from build123d import *

# Parameters (mm, degrees)
SKETCH1_R           = 3.175
BOSS_EXTRUDE1_DEPTH = 1.5875
FILLET1_R           = 9.525


with BuildPart() as part:
    # Sketch1 → Boss-Extrude1 (new body)
    with BuildSketch(Plane(origin=(0, 0, 0), x_dir=(1, 0, 0), z_dir=(0, 1, 0))):
        Polygon((12.7, 12.7), (14.2875, 12.7), (20.6375, 12.7), (22.225, 12.7), (47.625, 12.7), (47.625, -12.7), (22.225, -12.7), (12.7, -12.7), (-12.7, -12.7), (-22.225, -12.7), (-47.625, -12.7), (-47.625, 12.7), (-22.225, 12.7), (-12.7, 12.7), (-12.7, 25.4), (-12.7, 26.9875), (-14.2875, 26.9875), (-39.6875, 26.9875), (-39.6875, 77.7875), (-14.2875, 77.7875), (-12.7, 77.7875), (-12.7, 103.1875), (12.7, 103.1875), (12.7, 77.7875), (14.2875, 77.7875), (39.6875, 77.7875), (39.6875, 26.9875), (14.2875, 26.9875), (12.7, 26.9875), (12.7, 25.4), align=None)
        with Locations((26.9875, 36.5125)):
            Circle(SKETCH1_R, mode=Mode.SUBTRACT)
        with Locations((26.9875, 68.2625)):
            Circle(SKETCH1_R, mode=Mode.SUBTRACT)
        with Locations((0, 90.4875)):
            Circle(SKETCH1_R, mode=Mode.SUBTRACT)
        with Locations((34.925, 0)):
            Circle(SKETCH1_R, mode=Mode.SUBTRACT)
        Circle(SKETCH1_R, mode=Mode.SUBTRACT)
        with Locations((-34.925, 0)):
            Circle(SKETCH1_R, mode=Mode.SUBTRACT)
        with Locations((-26.9875, 68.2625)):
            Circle(SKETCH1_R, mode=Mode.SUBTRACT)
        with Locations((-26.9875, 36.5125)):
            Circle(SKETCH1_R, mode=Mode.SUBTRACT)
    extrude(amount=BOSS_EXTRUDE1_DEPTH)

    # Fillet1
    fillet1_edges = [part.edges().sort_by_distance(p)[0] for p in [
        (47.625, 0.79375, -12.7),
        (47.625, 0.79375, 12.7),
        (-47.625, 0.79375, 12.7),
        (-47.625, 0.79375, -12.7),
        (-39.6875, 0.79375, -26.9875),
        (-39.6875, 0.79375, -77.7875),
        (-12.7, 0.79375, -103.1875),
        (12.7, 0.79375, -103.1875),
        (39.6875, 0.79375, -77.7875),
        (39.6875, 0.79375, -26.9875),
    ]]
    fillet(fillet1_edges, radius=FILLET1_R)


solid = part.part
Read the model definition and answer for the solid it produces. Units are mm, in the model's axes. A direction names the side the tool comes from. Coordinates: 2 decimals unless noted, no trailing zeros. Loops run counter-clockwise (first coordinate to the right, second up) from the corner with the lowest first, then second, coordinate; pieces in that order, holes last. Notation, with made-up numbers: (-32.5, 63.5) -> (1.5, 63.5) arc R26 ccw to (1.5, 98.5) -> close; hole circle Ø9 at (-6.5, 53). An arc over 180 degrees is marked (long way). Answer in a Markdown table with one row per item.
Item 1: Each of these flat-tipped pins is pushed along its axis until it touches: P1, Ø0.8, axis at y = 0.5, z = -85, coming from the +X side; P2, Ø0.8, axis at x = -19, y = 1, coming from the -Z side; P3, Ø4, axis at x = -26.99, z = -68.26, coming from the +Y side; P4, Ø0.8, axis at y = 1, z = -17.5, coming from the -X side. Where does it stop, or does it pass through?
Returned:
| item | result |
|---|---|
| P1 | stops at x = 12.7 |
| P2 | stops at z = -77.79 |
| P3 | passes through |
| P4 | stops at x = -12.7 |
Item 2: A cutting plane is placed at D-D on z = -92. Determine the outline of the cut face in (x, y), plus the area to 3 significant figures.
Returned:
| item | result |
|---|---|
| outline | (-12.7, 0) -> (-2.79, 0) -> (-2.79, 1.59) -> (-12.7, 1.59) -> close; (2.79, 0) -> (12.7, 0) -> (12.7, 1.59) -> (2.79, 1.59) -> close |
| area | 31.5 mm^2 |
Item 3: A cutting plane is placed at B-B on z = 0. Give the number of separate pieces and of enclosed holes in the cut face, plus the area to 3 significant figures.
Returned:
| item | result |
|---|---|
| separate pieces | 4 |
| enclosed holes | 0 |
| area | 121 mm^2 |
Item 4: For a pull along X with two mould halves and no side action, classify faces 3 (the cylindrical face through (36.82, 0.8, -29.7)), 4 (the cylindrical face through (37.953, 0.783, -0.954)), 5 (the cylindrical face through (-36.971, 0.805, -74.923)) as released by +X, released by -X, zero draft, split by the parting line, or undercut.
Returned:
| item | result |
|---|---|
| face 3 | released by +X |
| face 4 | undercut |
| face 5 | released by -X |
Item 5: A cutting plane is placed at A-A on x = 0. Determine the outline of the cut face in (y, z) (1 decimal).
Returned:
| item | result |
|---|---|
| outline | (0, -103.2) -> (1.6, -103.2) -> (1.6, -93.7) -> (0, -93.7) -> close; (0, -87.3) -> (1.6, -87.3) -> (1.6, -3.2) -> (0, -3.2) -> close; (0, 3.2) -> (1.6, 3.2) -> (1.6, 12.7) -> (0, 12.7) -> close |
Item 6: Straight lines are drawn through the part: line 1 along X through (y, z) = (0.9, 0) (3 decimals); line 2 along X through (y, z) = (0.1, -71); line 3 along Z through (x, y) = (-30.5, 1.2). For each, find the intervals that lie inside material, in ascending order. Write a range as [from, to].
Returned:
| item | result |
|---|---|
| line 1 | x = [-47.625, -38.1], [-31.75, -3.175], [3.175, 31.75], [38.1, 47.625] |
| line 2 | x = [-39.29, -28.6], [-25.38, 25.38], [28.6, 39.29] |
| line 3 | z = [-77.78, -26.99], [-12.7, 12.7] |
Item 7: For faces 1 (the cylindrical face through (-0.69, 0.78, 3.1)), 2 (the cylindrical face through (-36.82, 0.8, -29.7)), determine the directions among +Z, -Z, +X, -X, +Y, -Y from which every point of the face is accessible in a straight line to the end or side of a thin tool.
Returned:
| item | result |
|---|---|
| face 1 | +Y, -Y |
| face 2 | -X, +Y, -Y |
